Build history of the part. All positions in model axes, mm. A direction names the side the tool comes from. Give positions to 0.01 mm unless a question says otherwise; leave off trailing zeros. Order: outer loops, then holes, each group sorted by start corner. A loop starts at its lowest first (then second) coordinate and runs counter-clockwise, first axis right, second up. Notation, with made-up numbers: (2, -24) -> (38, -24) arc R23 cw to (38, 6) -> close; hole circle Ø11 at (54.25, 27.5). An arc over 180 degrees is marked (long way). One line per item, written item: value. Start each with the question number.
(1) Two-plate mould, pull along Y, no slides. Class faces 1 (the flat face through (182, -1, 93)), 2 (the flat face through (194, -53, 93)), 3 (the cylindrical face through (190.12, -12.99, 92.52)): +Y half, -Y half, draft (parallel to the pull), parting line (faces both ways), or undercut.
(2) Which spindle directions (+Z, -Z, +X, -X, +Y, -Y) get a long thin tool onto all of the face, cutting with end or side? Do faces 4 (the cylindrical face through (189.07, 36.85, 92.52)), 5 (the flat face through (186, -40, 87.8)), 6 (the cylindrical face through (184, 30, 50)). Say none if no direction does.
(3) Saw through at A-A on y = -50.5. Give the cut face in (x, z), plus the area to 3 significant figures.
(4) Probe line 1 (Y direction, x = 186.5, z = 51); line 2 (Y direction, x = 187, z = 50); line 3 (X direction, y = -42, z = 92). List the from-to ranges inside material, lowest first.
(5) Saw through at C-C on z = 61.5. Give the cut face in (x, y).
(6) Saw through at D-D on x = 216.5. Give the cut face in (y, z).
(7) Saw through at B-B on y = 2.5. Give the cut face in (x, z), plus the area to 3 significant figures.
(8) Pin check, flat tips, straight feed: pin 1 (4.5 mm diameter, centred on x = 209, y = 13.5, fed in from -Z); pin 2 (2 mm diameter, centred on x = 191, y = 26.5, fed in from +Z); pin 3 (5 mm diameter, centred on y = 41, z = 58.5, fed in from +X); pin 4 (6 mm diameter, centred on x = 216.5, z = 75, fed in from +Y). Stop position of each tip, or through.
```python
from build123d import *

# Parameters (mm, degrees)
MAIN_PROFILE_SKETCH_R     = 1.7
MAIN_EXTRUSION_DEPTH      = 3
DETAIL_PROFILE_2_SKETCH_R = 3
DETAIL_EXTRUSION_2_DEPTH  = 3.2
DETAIL_PROFILE_3_SKETCH_R = 3
DETAIL_EXTRUSION_3_DEPTH  = 36.3
DETAIL_PROFILE_4_SKETCH_R = 1.7
DETAIL_EXTRUSION_4_DEPTH  = 3


with BuildPart() as part:
    # Main Profile Sketch → Main Extrusion (new body)
    with BuildSketch(Plane.XY.offset(94)):
        with BuildLine():
            Line((182, 53), (205.213560822, 53))
            ThreePointArc((205.213560822, 53), (210, 45.1), (214.786439178, 53))
            Line((214.786439178, 53), (218, 53))
            Line((218, 53), (218, -53))
            Line((218, -53), (214.786439178, -53))
            ThreePointArc((214.786439178, -53), (210, -45.1), (205.213560822, -53))
            Line((205.213560822, -53), (182, -53))
            Line((182, -53), (182, 53))
        make_face()
        with Locations((188.5, -40.5)):
            Circle(MAIN_PROFILE_SKETCH_R, mode=Mode.SUBTRACT)
        with Locations((188.5, -24.5)):
            Circle(MAIN_PROFILE_SKETCH_R, mode=Mode.SUBTRACT)
        with Locations((188.5, -13.5)):
            Circle(MAIN_PROFILE_SKETCH_R, mode=Mode.SUBTRACT)
        with Locations((211.5, -40.5)):
            Circle(MAIN_PROFILE_SKETCH_R, mode=Mode.SUBTRACT)
        with Locations((211.5, -24.5)):
            Circle(MAIN_PROFILE_SKETCH_R, mode=Mode.SUBTRACT)
        with Locations((211.5, -13.5)):
            Circle(MAIN_PROFILE_SKETCH_R, mode=Mode.SUBTRACT)
        with Locations((188.5, 2.5)):
            Circle(MAIN_PROFILE_SKETCH_R, mode=Mode.SUBTRACT)
        with Locations((191, 13.5)):
            Circle(MAIN_PROFILE_SKETCH_R, mode=Mode.SUBTRACT)
        with Locations((187.5, 37.5)):
            Circle(MAIN_PROFILE_SKETCH_R, mode=Mode.SUBTRACT)
        with Locations((187.5, 46.5)):
            Circle(MAIN_PROFILE_SKETCH_R, mode=Mode.SUBTRACT)
        with Locations((191, 26.5)):
            Circle(MAIN_PROFILE_SKETCH_R, mode=Mode.SUBTRACT)
        with Locations((211.5, 2.5)):
            Circle(MAIN_PROFILE_SKETCH_R, mode=Mode.SUBTRACT)
        with Locations((209, 13.5)):
            Circle(MAIN_PROFILE_SKETCH_R, mode=Mode.SUBTRACT)
        with Locations((200.5, 37.5)):
            Circle(MAIN_PROFILE_SKETCH_R, mode=Mode.SUBTRACT)
        with Locations((200.5, 46.5)):
            Circle(MAIN_PROFILE_SKETCH_R, mode=Mode.SUBTRACT)
        with Locations((209, 26.5)):
            Circle(MAIN_PROFILE_SKETCH_R, mode=Mode.SUBTRACT)
    extrude(amount=-MAIN_EXTRUSION_DEPTH)

    # Detail Profile 2 Sketch → Detail Extrusion 2 (add)
    with BuildSketch(Plane.XY.offset(91)):
        with Locations((216, 40)):
            Circle(DETAIL_PROFILE_2_SKETCH_R)
        with BuildLine():
            ThreePointArc((186.879170519, 40.842838727), (184.733306198, 39.476209859), (184.136505156, 37.003107219))
            ThreePointArc((184.136505156, 37.003107219), (181.558799586, 41.743714581), (186.879170519, 40.842838727))
        make_face()
        with BuildLine():
            ThreePointArc((186.217803802, -37.979765782), (185.120795302, -40.124532811), (185.720244978, -42.457795194))
            ThreePointArc((185.720244978, -42.457795194), (181.018348796, -39.668705422), (186.217803802, -37.979765782))
        make_face()
        with BuildLine():
            ThreePointArc((214.279755022, -42.457795194), (214.879204698, -40.124532811), (213.782196198, -37.979765782))
            ThreePointArc((213.782196198, -37.979765782), (218.981651204, -39.668705422), (214.279755022, -42.457795194))
        make_face()
    extrude(amount=-DETAIL_EXTRUSION_2_DEPTH)

    # Detail Profile 3 Sketch → Detail Extrusion 3 (add)
    with BuildSketch(Plane.XY.offset(87.8)):
        with Locations((216, 40)):
            Circle(DETAIL_PROFILE_3_SKETCH_R)
        with BuildLine():
            ThreePointArc((186.852864262, 39.072009967), (186.116653099, 38.488104929), (185.803081684, 37.602314357))
            ThreePointArc((185.803081684, 37.602314357), (181.558799586, 41.743714581), (186.852864262, 39.072009967))
        make_face()
        with BuildLine():
            ThreePointArc((186.98730258, -39.724276779), (186.810397651, -40.312266406), (186.853916932, -40.924747611))
            ThreePointArc((186.853916932, -40.924747611), (181.018348796, -39.668705422), (186.98730258, -39.724276779))
        make_face()
        with BuildLine():
            ThreePointArc((213.146083068, -40.924747611), (213.189602349, -40.312266406), (213.01269742, -39.724276779))
            ThreePointArc((213.01269742, -39.724276779), (218.981651204, -39.668705422), (213.146083068, -40.924747611))
        make_face()
    extrude(amount=-DETAIL_EXTRUSION_3_DEPTH)

    # Detail Profile 4 Sketch → Detail Extrusion 4 (add)
    # profile 1 of 4: a face of its own
    with BuildSketch(Plane.XY.offset(51.5)):
        with BuildLine():
            ThreePointArc((188.799011897, 38.596616656), (185.943513385, 38.18362959), (187.571358812, 35.801498331))
            ThreePointArc((187.571358812, 35.801498331), (183.73974082, 30.008475835), (180.692810861, 36.25))
            ThreePointArc((180.692810861, 36.25), (182.609663272, 44.802807906), (188.799011897, 38.596616656))
        make_face()
        with Locations((184, 34)):
            Circle(DETAIL_PROFILE_4_SKETCH_R, mode=Mode.SUBTRACT)
    # profile 2 of 4: a face of its own
    with BuildSketch(Plane.XY.offset(51.5)):
        with BuildLine():
            ThreePointArc((188.863411368, -38.839297685), (186.810397651, -40.312266406), (188.490003266, -42.199970607))
            ThreePointArc((188.490003266, -42.199970607), (180.96680039, -43.974883662), (180.692810861, -36.25))
            ThreePointArc((180.692810861, -36.25), (184, -30), (187.307189139, -36.25))
            ThreePointArc((187.307189139, -36.25), (188.285533081, -37.424304713), (188.863411368, -38.839297685))
        make_face()
        with Locations((184, -34)):
            Circle(DETAIL_PROFILE_4_SKETCH_R, mode=Mode.SUBTRACT)
    # profile 3 of 4: a face of its own
    with BuildSketch(Plane.XY.offset(51.5)):
        with BuildLine():
            ThreePointArc((211.509996734, -42.199970607), (213.189602349, -40.312266406), (211.136588632, -38.839297685))
            ThreePointArc((211.136588632, -38.839297685), (211.714466919, -37.424304713), (212.692810861, -36.25))
            ThreePointArc((212.692810861, -36.25), (216, -30), (219.307189139, -36.25))
            ThreePointArc((219.307189139, -36.25), (219.03319961, -43.974883662), (211.509996734, -42.199970607))
        make_face()
        with Locations((216, -34)):
            Circle(DETAIL_PROFILE_4_SKETCH_R, mode=Mode.SUBTRACT)
    # profile 4 of 4: a face of its own
    with BuildSketch(Plane.XY.offset(51.5)):
        with BuildLine():
            ThreePointArc((212.692810861, 36.25), (216, 30), (219.307189139, 36.25))
            ThreePointArc((219.307189139, 36.25), (216, 45), (212.692810861, 36.25))
        make_face()
        with Locations((216, 34)):
            Circle(DETAIL_PROFILE_4_SKETCH_R, mode=Mode.SUBTRACT)
    extrude(amount=-DETAIL_EXTRUSION_4_DEPTH)


solid = part.part
```
Results below:
1. face 1: draft
1. face 2: -Y half
1. face 3: undercut
2. face 4: +Z, -Z
2. face 5: none
2. face 6: -Z
3. outline: (182, 91) -> (204.6, 91) -> (204.6, 94) -> (182, 94) -> close; (215.4, 91) -> (218, 91) -> (218, 94) -> (215.4, 94) -> close
3. area: 75.6 mm²
4. line 1: y = -44.33 to -30.88, 30.88 to 36.13, 38.87 to 44.33
4. line 2: y = -44 to -41.3, -39.7 to -31.35, 31.35 to 35.88, 39.12 to 44
4. line 3: x = 182 to 187.7, 189.3 to 210.7, 212.3 to 218
5. outline: (185.8, 37.6) arc R1.7 cw to (186.85, 39.07) arc R3 ccw (long way) to start; (186.85, -40.92) arc R1.7 cw to (186.99, -39.72) arc R3 ccw (long way) to start; circle Ø6 at (216, 40); (213.01, -39.72) arc R1.7 cw to (213.15, -40.92) arc R3 ccw (long way) to start
6. outline: (-53, 91) -> (-42.96, 91) -> (-42.96, 51.5) -> (-44.97, 51.5) -> (-44.97, 48.5) -> (-35.62, 48.5) -> (-35.62, 51.5) -> (-37.04, 51.5) -> (-37.04, 91) -> (37.04, 91) -> (37.04, 51.5) -> (35.62, 51.5) -> (35.62, 48.5) -> (44.97, 48.5) -> (44.97, 51.5) -> (42.96, 51.5) -> (42.96, 91) -> (53, 91) -> (53, 94) -> (-53, 94) -> close; (-32.38, 48.5) -> (-30.03, 48.5) -> (-30.03, 51.5) -> (-32.38, 51.5) -> close; (30.03, 48.5) -> (32.38, 48.5) -> (32.38, 51.5) -> (30.03, 51.5) -> close
7. outline: (182, 91) -> (186.8, 91) -> (186.8, 94) -> (182, 94) -> close; (190.2, 91) -> (209.8, 91) -> (209.8, 94) -> (190.2, 94) -> close; (213.2, 91) -> (218, 91) -> (218, 94) -> (213.2, 94) -> close
7. area: 87.6 mm²
8. pin 1: stops at z = 91
8. pin 2: passes through
8. pin 3: stops at x = 219
8. pin 4: stops at y = 43
